Source: CAD feature listing. Evaluate the final solid. Frame: model axes, mm. A direction names the side the tool comes from. Coordinates: 2 decimals unless noted, no trailing zeros. Order: outer loops, then holes, each group sorted by start corner. A loop starts at its lowest first (then second) coordinate and runs counter-clockwise, first axis right, second up.
```python
from build123d import *

# Parameters (mm, degrees)
F0_W          = 98.744937
F0_H          = 66.599365
F1_DEPTH      = 76.2
F4_DEPTH      = 12.7
F5_R          = 24.638622
F6_DEPTH      = 12.7
F6_DEPTH_BACK = 88.9
F7_R          = 6.776006
F7_R_2        = 6.130863
F8_DEPTH      = 66.600365
F10_DEPTH     = 12.7


with BuildPart() as f1:
    # F0 (on Front) → F1 (new body)
    with BuildSketch(Plane.XZ):
        with Locations((-17.064217, -16.306898)):
            Rectangle(F0_W, F0_H)
    extrude(amount=-F1_DEPTH)

    # F3 (on face) → F4 (join)
    with BuildSketch(Plane.XZ):
        with BuildLine():
            ThreePointArc((12.440301, 16.913241), (-12.653938, -7.34435), (-37.748177, 16.913241))
            Line((-37.748177, 16.913241), (-47.070116, 16.913241))
            ThreePointArc((-47.070116, 16.913241), (-13.344199, -17.828973), (20.381717, 16.913241))
            Line((20.381717, 16.913241), (12.440301, 16.913241))
        make_face()
    extrude(amount=F4_DEPTH)

    # F5 (on Front) → F6 (cut, two sides)
    with BuildSketch(Plane.XZ) as f6_sk:
        with Locations((-12.513756, 17.087433)):
            Circle(F5_R)
    extrude(amount=F6_DEPTH, mode=Mode.SUBTRACT)
    extrude(f6_sk.sketch, amount=-F6_DEPTH_BACK, mode=Mode.SUBTRACT)

    # F7 (on face) → F8 (cut, through all)
    with BuildSketch(Plane.XY.offset(16.992785)):
        with Locations((23.502037, 37.125945)):
            Circle(F7_R)
        with Locations((-51.750846, 38.397469)):
            Circle(F7_R_2)
    extrude(amount=-F8_DEPTH, mode=Mode.SUBTRACT)

    # F9 (on face) → F10 (join)
    with BuildSketch(Plane(origin=(0, 76.2, 0), x_dir=(-1, 0, 0), z_dir=(0, 1, 0))):
        with BuildLine():
            ThreePointArc((37.152196, 16.992785), (12.513756, -8.492675), (-12.124685, 16.992785))
            Line((-12.124685, 16.992785), (-22.216468, 16.992785))
            ThreePointArc((-22.216468, 16.992785), (12.40618, -17.061067), (47.028828, 16.992785))
            Line((47.028828, 16.992785), (37.152196, 16.992785))
        make_face()
    extrude(amount=F10_DEPTH)


solid = f1.part
```
Q1. Set-up query: faces 1 (the flat face through (-18, 76.2, -23)), 2 (the cylindrical face through (11.405, -6.261, 10.581)), 3 (the flat face through (-14, -12.7, -8)). Return all of +Z, -Z, +X, -X, +Y, -Y with unobstructed straight access to the full face (end or side cutting, diameter ignored); none if empty.
Solutions:
face 1: -Z, +Y
face 2: +Z, -Y
face 3: +Z, -Z, +X, -X, -Y
Q2. Pin query (flat end, axial travel): P1, Ø4.5, axis at x = -41, y = -5, coming from the +Z side; P2, Ø1, axis at x = -34.5, y = 66.5, coming from the +Z side; P3, Ø5, axis at x = -53.5, z = -4, coming from the +Y side. Return the tip coordinate at first contact, or that it passes through.
Solutions:
P1: stops at z = 16.91
P2: stops at z = 7.02
P3: stops at y = 76.2
Q3. Section query C-C on y = 47.5. Output: boundary loops of the cut face in (x, z), plus the area to 3 significant figures.
Solutions:
outline: (-66.44, -49.61) - (32.31, -49.61) - (32.31, 16.99) - (12.12, 16.99) arc R24.64 cw to (-37.15, 16.99) - (-66.44, 16.99) - close
area: 5,630 mm2
Q4. Pull-direction query (X, two-part tool) for faces 4 (the cylindrical face through (-34.634, -6.261, 5.627)), 5 (the flat face through (-42, -6, 16.913)), 6 (the cylindrical face through (-11.653, 82.461, -17.053)), 7 (the flat face through (-66.437, 38, -17)); classes: pulls with the +X half, pulls with the -X half, needs draft (parallel to the pull), parting line crosses it, or undercut.
Solutions:
face 4: undercut
face 5: needs draft
face 6: parting line crosses it
face 7: pulls with the -X half
Q5. Section query A-A on x = 26. Output: boundary loops of the cut face in (y, z).
Solutions:
outline: (0, -49.61) - (30.83, -49.61) - (30.83, 16.99) - (0, 16.99) - close; (43.42, -49.61) - (76.2, -49.61) - (76.2, 16.99) - (43.42, 16.99) - close
Q6. Section query B-B on z = -11.5. Output: boundary loops of the cut face in (x, y), plus the area to 3 significant figures.
Solutions:
outline: (-66.44, 0) - (-33.02, 0) - (-33.02, -12.7) - (6.33, -12.7) - (6.33, 0) - (32.31, 0) - (32.31, 76.2) - (6.41, 76.2) - (6.41, 88.9) - (-31.23, 88.9) - (-31.23, 76.2) - (-66.44, 76.2) - close; hole circle Ø12.26 at (-51.75, 38.4); hole circle Ø13.55 at (23.5, 37.13)
area: 8,240 mm2
Q7. Material intervals for line 1 along X through (y, z) = (43, -18); line 2 along X through (y, z) = (37, 13.5); line 3 along Z through (x, y) = (-12, 27), sorted ascending.
Solutions:
line 1: x = -66.44 to -55.8, -47.7 to 20.12, 26.88 to 32.31
line 2: x = -66.44 to -57.72, -45.78 to -36.89, 11.86 to 16.73, 30.28 to 32.31
line 3: z = -49.61 to -7.55
Q8. Section query D-D on x = -11.5. Output: boundary loops of the cut face in (y, z).
Solutions:
outline: (-12.7, -17.78) - (0, -17.78) - (0, -49.61) - (76.2, -49.61) - (76.2, -17.05) - (88.9, -17.05) - (88.9, -8.47) - (76.2, -8.47) - (76.2, -7.53) - (-12.7, -7.53) - close
